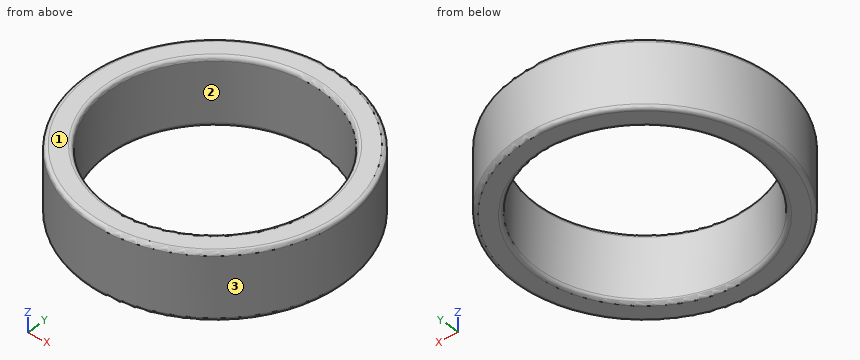
from build123d import *

# Parameters (mm, degrees)
F0_R     = 13.5
F0_R_2   = 11.1
F1_DEPTH = 7
F2_R     = 0.4


# Not quite as in the source:
# - a feature names something its author has since deleted; it is built from what else it names


with BuildPart() as f1:
    # F0 (on Top) → F1 (new body)
    with BuildSketch(Plane.XY):
        Circle(F0_R)
        Circle(F0_R_2, mode=Mode.SUBTRACT)
    extrude(amount=F1_DEPTH)

    # F2
    f2_edges = [f1.edges().sort_by_distance(p)[0] for p in [
        (-11.1, 0, 7),
        (-13.5, 0, 7),
        (-13.5, 0, 0),
        (-11.1, 0, 0),
    ]]
    fillet(f2_edges, radius=F2_R)


solid = f1.part
Check sheet for the modelled part. Datum: model origin and axes. Units: mm. Face numbers are marked on the shaded views. Round coordinates to 2 decimals unless told otherwise and drop trailing zeros. Order: outer loops, then holes, each group sorted by start corner. A loop starts at its lowest first (then second) coordinate and runs counter-clockwise, first axis right, second up.
(1) Draft check along Y on the marked faces 1, 2 and 3. Enter one of: pulls with the +Y half, pulls with the -Y half, needs draft (parallel to the pull), parting line crosses it, or undercut.
(2) Go/stop test with flat-tipped pins: P1, Ø4, axis at x = 3, z = 4, coming from the -Y side; P2, Ø6, axis at x = -5.5, y = -2, coming from the +Z side; P3, Ø4, axis at y = 2.5, z = 4, coming from the +X side; P4, Ø1, axis at y = 2, z = 2, coming from the -X side. Record where each tip stops, or that it passes through.
(3) Cross-section at A-A, the plane y = 0. Enter the section's corners in (x, z).
(4) Scan lines: probe 1 along Y at (x, z) = (0, 2); probe 2 along X at (y, z) = (6, 5.75); probe 3 along X at (y, z) = (-8.25, 4.5). Record each from-to range of solid material in increasing order.
(5) Cross-section at C-C, the plane z = 1.75. Enter the section's corners in (x, y), and give its area (3 significant figures).
Check sheet entries:
1. face 1: needs draft
1. face 2: undercut
1. face 3: parting line crosses it
2. P1: stops at y = -13.46
2. P2: passes through
2. P3: stops at x = 13.49
2. P4: stops at x = -13.42
3. outline: (-13.5, 0.4) arc R0.4 ccw to (-13.1, 0) - (-11.5, 0) arc R0.4 ccw to (-11.1, 0.4) - (-11.1, 6.6) arc R0.4 ccw to (-11.5, 7) - (-13.1, 7) arc R0.4 ccw to (-13.5, 6.6) - close; (11.1, 0.4) arc R0.4 ccw to (11.5, 0) - (13.1, 0) arc R0.4 ccw to (13.5, 0.4) - (13.5, 6.6) arc R0.4 ccw to (13.1, 7) - (11.5, 7) arc R0.4 ccw to (11.1, 6.6) - close
4. probe 1: y = -13.5 to -11.1, 11.1 to 13.5
4. probe 2: x = -12.09 to -9.34, 9.34 to 12.09
4. probe 3: x = -10.69 to -7.43, 7.43 to 10.69
5. outline: circle Ø27 at (0, 0); hole circle Ø22.2 at (0, 0)
5. area: 185 mm2
